Part model, mm, in its own coordinate system. A direction names the side the tool comes from. Round coordinates to 2 decimals unless told otherwise and drop trailing zeros. Order: outer loops, then holes, each group sorted by start corner. A loop starts at its lowest first (then second) coordinate and runs counter-clockwise, first axis right, second up. Notation, with made-up numbers: (0.25, 58) -> (36.25, 58) arc R8 cw to (36.25, 66) -> close; hole circle Ø5 at (54, 28.25). An arc over 180 degrees is marked (long way). Answer as a JSON object with one key per item and string values. Group by question number.
```python
from build123d import *

# Parameters (mm, degrees)
F3_DEPTH = 3
F4_R     = 9
F5_DEPTH = 1.5


with BuildPart() as f1:
    # F0 (on Front) → F1 (revolve)
    with BuildSketch(Plane.XZ):
        with BuildLine():
            Line((-4, 0), (0, 0))
            Line((0, 0), (0, 44))
            Line((0, 44), (-3.5, 44))
            ThreePointArc((-3.5, 44), (-5.650581, 43.310814), (-7, 41.5))
            Line((-7, 41.5), (-7, 40))
            Line((-7, 40), (-4, 40))
            Line((-4, 40), (-4, 0))
        make_face()
    revolve(axis=Axis((0, 0, 22), (0, 0, 1)))

    # F2 (on face) → F3 (cut)
    with BuildSketch(Plane.XY.offset(44)):
        Polygon((1.443376, 2.5), (-1.443376, 2.5), (-2.886751, 0), (-1.443376, -2.5), (1.443376, -2.5), (2.886751, 0), align=None)
    extrude(amount=-F3_DEPTH, mode=Mode.SUBTRACT)

    # F4 (on face) → F5 (join)
    with BuildSketch(Plane(origin=(0, 0, 40), x_dir=(1, 0, 0), z_dir=(0, 0, -1))):
        Circle(F4_R)
    extrude(amount=-F5_DEPTH)


solid = f1.part
```
Q1. Band-saw the part on B-B (y = 7.5). List the corners of the cut face in (x, z).
Q2. Drop flat-ended pins along their axis: pin 1 Ø4 at (x, y) = (5, -3.5) entering from +Z; pin 2 Ø9 at (x, y) = (-1, -0.5) entering from +Z; pin 3 Ø8 at (x, z) = (-0.5, 30.5) entering from +Y; pin 4 Ø10 at (y, z) = (-5.5, 27) entering from +X. Give the stop position or say it passes through.
Q3. Wall check: line 1 (Z direction, x = -4.75, y = -5.25); line 2 (Z direction, x = 0.5, y = -2); line 3 (X direction, y = 0.25, z = 19.5). Give the ranges that are in metal, low to high. Write a range as [from, to].
Q4. Band-saw the part on A-A (z = 28). List the corners of the cut face in (x, y), plus the area to 3 significant figures.
Q5. Two-plate mould, pull along X, no slides. Class faces 4 (the flat face through (2.155, -1.267, 42.768)), 5 (the cylindrical face through (-1.172, -8.923, 40.74)), 6 (the flat face through (-2, 2, 44)): +X half, -X half, draft (parallel to the pull), parting line (faces both ways), or undercut.
Q6. Which spindle directions (+Z, -Z, +X, -X, +Y, -Y) get a long thin tool onto all of the face, cutting with end or side? Do faces 1 (the flat face through (2.175, 1.233, 42.768)), 2 (the flat face through (0, 0, 0)), 3 (the cylindrical face through (0.867, 3.905, 19.72)). Say none if no direction does.
Completed:
{
 "1": {"outline": "(-4.97, 40) -> (4.97, 40) -> (4.97, 41.5) -> (-4.97, 41.5) -> close"},
 "2": {"pin 1": "z = 43.95", "pin 2": "z = 44", "pin 3": "y = 4", "pin 4": "x = 3.97"},
 "3": {"line 1": "[40, 41.5]", "line 2": "[0, 41.5]", "line 3": "[-3.99, 3.99]"},
 "4": {"outline": "circle Ø8 at (0, 0)", "area": "50.3 mm2"},
 "5": {"face 4": "undercut", "face 5": "parting line", "face 6": "draft"},
 "6": {"face 1": "+Z", "face 2": "-Z, +X, -X, +Y, -Y", "face 3": "-Z"}
}
